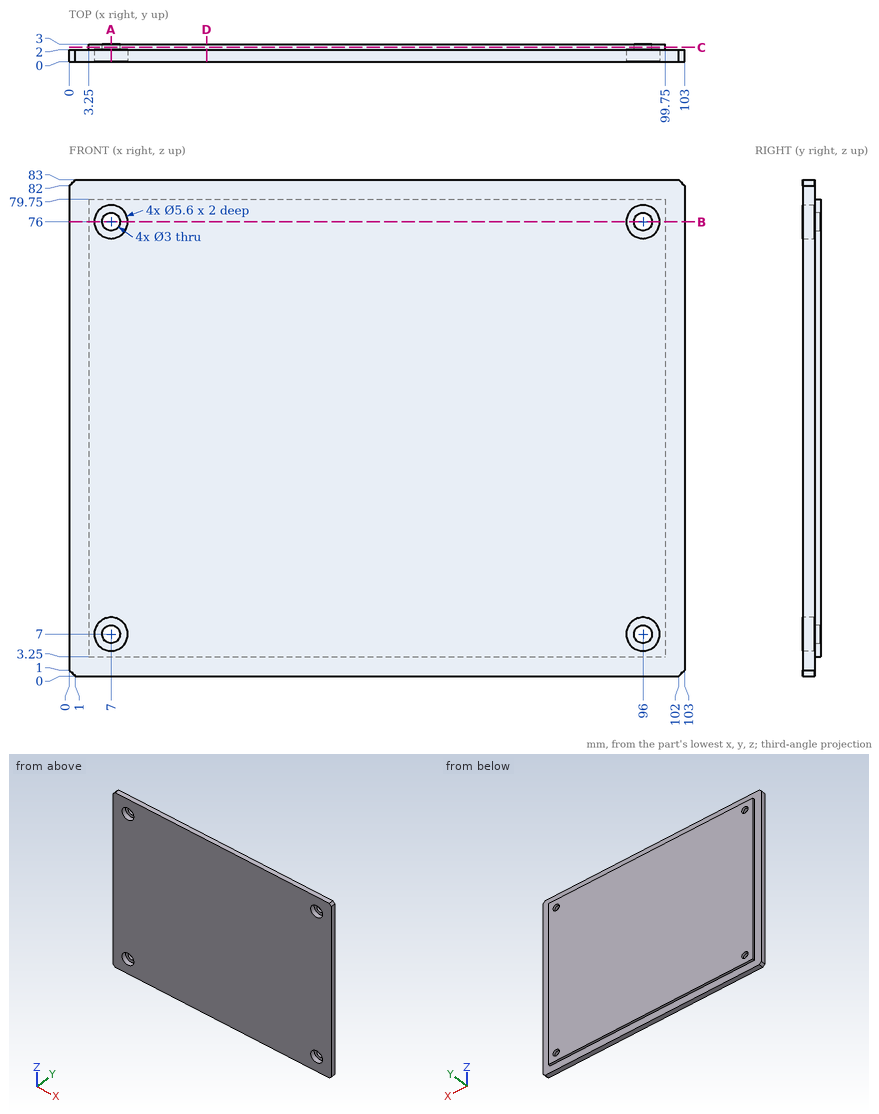
Geometry check sheet. Reference: drawing and pictorial views, mm from the part's lowest x, y, z. Give positions to 0.01 mm unless a question says otherwise; leave off trailing zeros. Write each loop counter-clockwise with the first axis right and the second up, starting at its lowest first coordinate (ties: lowest second). Pieces come first, ordered by that corner, then holes. Notation, with made-up numbers: M 71,62.25 L 75,62.25 A22 cw 75,70.25 Z; hole C 53,89.5 d10. An arc over 180 degrees is marked long. Put each result on its own line as item: value. Start each with the question number.
1. Section check D-D (x = 23). Record the cut outline in (y, z).
2. Go/stop test with a flat-tipped pin: pin 1 Ø0.8 at (y, z) = (2.5, 39) entering from -X. Record where the tip stops, or that it passes through.
3. Scan lines: line 1 along X through (y, z) = (1.55, 7); line 2 along Z through (x, y) = (96, 2.35); line 3 along X through (y, z) = (2.85, 76). Record each from-to range of solid material in increasing order. Write a range as [from, to].
4. Section check C-C (y = 2.45). Record the cut outline in (x, z).
5. Section check A-A (x = 7). Record the cut outline in (y, z), and give its area (3 significant figures).
6. Section check B-B (z = 76). Record the cut outline in (x, y).
Answer list:
1. outline: M 0,0 L 2,0 L 2,3.25 L 3,3.25 L 3,79.75 L 2,79.75 L 2,83 L 0,83 Z
2. pin 1: x = 3.25
3. line 1: [0, 4.2], [9.8, 93.2], [98.8, 103]
3. line 2: [3.25, 5.5], [8.5, 74.5], [77.5, 79.75]
3. line 3: [3.25, 5.5], [8.5, 94.5], [97.5, 99.75]
4. outline: M 3.25,3.25 L 99.75,3.25 L 99.75,79.75 L 3.25,79.75 Z; hole C 7,7 d3; hole C 7,76 d3; hole C 96,7 d3; hole C 96,76 d3
5. outline: M 0,0 L 2,0 L 2,3.25 L 3,3.25 L 3,5.5 L 2,5.5 L 2,4.2 L 0,4.2 Z; M 0,9.8 L 2,9.8 L 2,8.5 L 3,8.5 L 3,74.5 L 2,74.5 L 2,73.2 L 0,73.2 Z; M 0,78.8 L 2,78.8 L 2,77.5 L 3,77.5 L 3,79.75 L 2,79.75 L 2,83 L 0,83 Z
5. area: 214 mm2
6. outline: M 0,0 L 4.2,0 L 4.2,2 L 5.5,2 L 5.5,3 L 3.25,3 L 3.25,2 L 0,2 Z; M 8.5,2 L 9.8,2 L 9.8,0 L 93.2,0 L 93.2,2 L 94.5,2 L 94.5,3 L 8.5,3 Z; M 97.5,2 L 98.8,2 L 98.8,0 L 103,0 L 103,2 L 99.75,2 L 99.75,3 L 97.5,3 Z
